Could you check a few things on this model? Use its own coordinates, in mm. Round coordinates to 2 decimals unless told otherwise and drop trailing zeros. Loops run counter-clockwise (first coordinate to the right, second up) from the corner with the lowest first, then second, coordinate; pieces in that order, holes last. Notation, with made-up numbers: (27.25, -37) -> (78.25, -37) arc R26 cw to (78.25, -19) -> close; hole circle Ø1 at (-3, 49). An arc over 180 degrees is marked (long way). One line per item, written item: value.
```python
from build123d import *

# Parameters (mm, degrees)
SKETCH1_R           = 20
BOSS_EXTRUDE1_DEPTH = 1.6
SKETCH2_R           = 0.743
CUT_EXTRUDE2_DEPTH  = 1.6


with BuildPart() as part:
    # Sketch1 → Boss-Extrude1 (new body)
    with BuildSketch(Plane(origin=(0, 0, 0), x_dir=(1, 0, 0), z_dir=(0, 1, 0))):
        Circle(SKETCH1_R)
    extrude(amount=-BOSS_EXTRUDE1_DEPTH)

    # Sketch2 → Cut-Extrude2 (cut)
    with BuildSketch(Plane.XZ.offset(1.6)):
        with Locations((-0.00171005, 12.498814086)):
            Circle(SKETCH2_R)
        with Locations((10.823435491, 6.25088799)):
            Circle(SKETCH2_R)
        with Locations((10.825145541, -6.247926096)):
            Circle(SKETCH2_R)
        with Locations((0.00171005, -12.498814086)):
            Circle(SKETCH2_R)
        with Locations((-10.823435491, -6.25088799)):
            Circle(SKETCH2_R)
    extrude(amount=-CUT_EXTRUDE2_DEPTH, mode=Mode.SUBTRACT)


solid = part.part
```
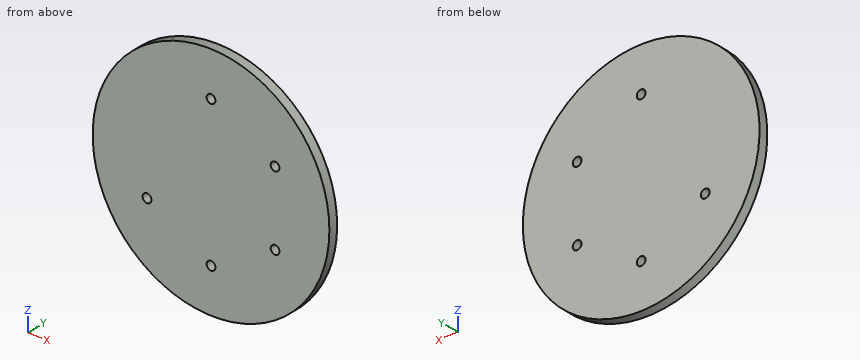
(1) Please list where these lines run through material, in increasing order: L1, parallel to Z at x = 0, y = -1.2; L2, parallel to Z at x = -6, y = -0.6; L3, parallel to Z at x = -7, y = -0.95 (3 decimals).
Results below:
L1: z = -20 to -13.24, -11.76 to 11.76, 13.24 to 20
L2: z = -19.08 to 19.08
L3: z = -18.735 to 18.735
(2) Imagine slicing it at A-A on x = 0. Write out the boundary of the cut face in (y, z).
Results below:
outline: (-1.6, -20) -> (0, -20) -> (0, -13.24) -> (-1.6, -13.24) -> close; (-1.6, -11.76) -> (0, -11.76) -> (0, 11.76) -> (-1.6, 11.76) -> close; (-1.6, 13.24) -> (0, 13.24) -> (0, 20) -> (-1.6, 20) -> close
(3) Imagine slicing it at B-B on y = -1.05. Write out the boundary of the cut face in (x, z), then the cut area to 3 significant figures.
Results below:
outline: circle Ø40 at (0, 0); hole circle Ø1.49 at (-10.82, -6.25); hole circle Ø1.49 at (0, -12.5); hole circle Ø1.49 at (0, 12.5); hole circle Ø1.49 at (10.83, -6.25); hole circle Ø1.49 at (10.82, 6.25)
area: 1,250 mm²
(4) Imagine slicing it at D-D on z = 4.5. Write out the boundary of the cut face in (x, y), then the cut area to 3 significant figures.
Results below:
outline: (-19.49, -1.6) -> (19.49, -1.6) -> (19.49, 0) -> (-19.49, 0) -> close
area: 62.4 mm²
(5) For pin 1 Ø1.2 at (x, z) = (-10.82, -6.25) entering from -Y, with a flat end and sliding along its axis, tell me the tip position at first contact or that it passes through.
Results below:
pin 1: passes through
(6) Imagine slicing it at C-C on x = 16. Write out the boundary of the cut face in (y, z), then the cut area to 3 significant figures.
Results below:
outline: (-1.6, -12) -> (0, -12) -> (0, 12) -> (-1.6, 12) -> close
area: 38.4 mm²
